Read the model definition and answer for the solid it produces. Units are mm, in the model's axes. A direction names the side the tool comes from. Coordinates: 2 decimals unless noted, no trailing zeros. Loops run counter-clockwise (first coordinate to the right, second up) from the corner with the lowest first, then second, coordinate; pieces in that order, holes last. Notation, with made-up numbers: (46.25, 58.25) -> (50.25, 58.25) arc R19 cw to (50.25, 68.25) -> close; hole circle Ø3 at (-33, 5.5). An arc over 180 degrees is marked (long way). Answer as a JSON object with one key per item and string values. Group by question number.
1) Which of the six approach directions +Z, -Z, +X, -X, +Y, -Y give full straight-line access (tool end or side, diameter ignored) to faces 4 (the face through (12, 11.683, 16)), 5 (the face through (-13, 0, 9)), 6 (the face through (1, -22.892, 10)), 7 (the face through (-4.535, -21, 12))?
2) Section A-A, the plane y = 21 is taken. Give the vertices of the cut face in (x, z).
3) Flat-ended cylindrical pins translate along their axes: P1, Ø4, axis at x = -2.5, y = 0.5, coming from the -Z side; P2, Ø1.5, axis at x = 3, z = 16.5, coming from the +Y side; P3, Ø1.5, axis at x = 8.5, y = 6.5, coming from the +Z side. Find the tip coordinate at first contact, or state that the pin passes through.
4) Determine the mould class of faces 1 (the face through (-14.14, -8.51, 18)), 2 (the face through (0, 29.892, 12)), 3 (the face through (16.253, -28.368, 13.437)) for opening direction Y: released by +Y, released by -Y, zero draft, split by the parting line, or undercut.
5) Section D-D, the plane x = 9 is taken. Give the vertices of the cut face in (y, z) (3 decimals), plus the area to 3 significant figures.
6) Section B-B, the plane x = 16.47 is taken. Give the vertices of the cut face in (y, z).
7) Consider probe 1 along Y at (x, z) = (16.47, 11.8); probe 2 along Y at (x, z) = (5.5, 10.75); probe 3 along Y at (x, z) = (12.5, 9.5) (3 decimals). Determine where each line is inside the solid, lowest interval first. Write a range as [from, to].
8) Section C-C, the plane x = 5 is taken. Give the vertices of the cut face in (y, z), plus the area to 3 significant figures.
from build123d import *

# Parameters (mm, degrees)
SKETCH002_W     = 37.94
SKETCH002_H     = 59.784
SKETCH002_R     = 1
SKETCH002_W_2   = 23.906
SKETCH002_H_2   = 8.634
SKETCH002_W_3   = 11.189
SKETCH002_H_3   = 6.022
SKETCH002_W_4   = 3.58
SKETCH002_H_4   = 8.639
SKETCH002_W_5   = 6.685
SKETCH002_H_5   = 4.785
SKETCH002_W_6   = 7.878
SKETCH002_H_6   = 5.832
PAD_DEPTH       = 9
SKETCH_W        = 27.94
SKETCH_H        = 36.575
SKETCH_H_2      = 12.209
POCKET_DEPTH    = 5
POCKET001_DEPTH = 37.94
SKETCH004_W     = 23.94
SKETCH004_H     = 45.784
POCKET002_DEPTH = 2
SKETCH005_W     = 23.94
SKETCH005_H     = 4
POCKET003_DEPTH = 5
FILLET_R        = 0.75


with BuildPart() as part:
    # Sketch002 → Pad (new body)
    with BuildSketch(Plane.XY.offset(9)):
        Rectangle(SKETCH002_W, SKETCH002_H)
        with Locations((-16.47, 27.392)):
            Circle(SKETCH002_R, mode=Mode.SUBTRACT)
        with Locations((16.47, 27.392)):
            Circle(SKETCH002_R, mode=Mode.SUBTRACT)
        with Locations((-16.47, -27.392)):
            Circle(SKETCH002_R, mode=Mode.SUBTRACT)
        with Locations((16.47, -27.392)):
            Circle(SKETCH002_R, mode=Mode.SUBTRACT)
        with Locations((-0.493, 18.53)):
            Rectangle(SKETCH002_W_2, SKETCH002_H_2, mode=Mode.SUBTRACT)
        with Locations((-2.4905, 7.679)):
            Rectangle(SKETCH002_W_3, SKETCH002_H_3, mode=Mode.SUBTRACT)
        with Locations((7.885, 7.8825)):
            Rectangle(SKETCH002_W_4, SKETCH002_H_4, mode=Mode.SUBTRACT)
        with Locations((9.428, -19.7805)):
            Rectangle(SKETCH002_W_4, SKETCH002_H_4, mode=Mode.SUBTRACT)
        with Locations((9.6625, -9.8675)):
            Rectangle(SKETCH002_W_5, SKETCH002_H_5, mode=Mode.SUBTRACT)
        with Locations((-8.6435, -14.9585)):
            Rectangle(SKETCH002_W_5, SKETCH002_H_5, mode=Mode.SUBTRACT)
        with Locations((-8.121, 1.626)):
            Rectangle(SKETCH002_W_6, SKETCH002_H_6, mode=Mode.SUBTRACT)
        with Locations((-8.474, -20.887)):
            Rectangle(SKETCH002_W_6, SKETCH002_H_6, mode=Mode.SUBTRACT)
    extrude(amount=PAD_DEPTH)

    # Sketch (on Face42 of Pad) → Pocket (cut)
    with BuildSketch(Plane.XY.offset(18)):
        with Locations((0, -6.6045)):
            Rectangle(SKETCH_W, SKETCH_H)
        with Locations((0, 18.7875)):
            Rectangle(SKETCH_W, SKETCH_H_2)
    extrude(amount=-POCKET_DEPTH, mode=Mode.SUBTRACT)

    # Sketch003 → Pocket001 (cut)
    with BuildSketch(Plane(origin=(18.97, 0, 9), x_dir=(0, 1, 0), z_dir=(1, 0, 0))):
        Polygon((12.683, 9), (29.892, 9), (29.892, 5.5), (16.183, 5.5), align=None)
    extrude(amount=-POCKET001_DEPTH, mode=Mode.SUBTRACT)

    # Sketch004 → Pocket002 (cut)
    with BuildSketch(Plane(origin=(0, 0, 9), x_dir=(1, 0, 0), z_dir=(0, 0, -1))):
        Rectangle(SKETCH004_W, SKETCH004_H)
    extrude(amount=-POCKET002_DEPTH, mode=Mode.SUBTRACT)

    # Sketch005 (on Face39 of Pocket002) → Pocket003 (cut)
    with BuildSketch(Plane.XY.offset(18)):
        with Locations((0, -26.892)):
            Rectangle(SKETCH005_W, SKETCH005_H)
    extrude(amount=-POCKET003_DEPTH, mode=Mode.SUBTRACT)

    # Fillet
    fillet_edges = [part.edges().sort_by_distance(p)[0] for p in [
        (-18.97, -29.892, 13.5),
        (18.97, -29.892, 13.5),
        (18.97, 29.892, 11.75),
        (-18.97, 29.892, 11.75),
    ]]
    fillet(fillet_edges, radius=FILLET_R)


solid = part.part
Determined:
{
 "1": {"face 4": "+Z", "face 5": "-Z, +X, -X, +Y, -Y", "face 6": "-Z", "face 7": "+Z, -Z"},
 "2": {"outline": "(-18.97, 9) -> (-12.45, 9) -> (-12.45, 13) -> (-13.97, 13) -> (-13.97, 14.5) -> (-18.97, 14.5) -> close; (11.46, 11) -> (11.97, 11) -> (11.97, 9) -> (18.97, 9) -> (18.97, 14.5) -> (13.97, 14.5) -> (13.97, 13) -> (11.46, 13) -> close"},
 "3": {"P1": "z = 11", "P2": "y = 12.68", "P3": "through"},
 "4": {"face 1": "zero draft", "face 2": "released by +Y", "face 3": "undercut"},
 "5": {"outline": "(-29.892, 9) -> (-24.1, 9) -> (-24.1, 13) -> (-28.892, 13) -> (-28.892, 18) -> (-29.892, 18) -> close; (-15.461, 11) -> (-12.26, 11) -> (-12.26, 13) -> (-15.461, 13) -> close; (-7.475, 11) -> (3.563, 11) -> (3.563, 13) -> (-7.475, 13) -> close; (12.202, 11) -> (14.213, 11) -> (14.213, 13) -> (12.683, 13) -> (12.683, 18) -> (12.202, 18) -> close; (22.847, 11) -> (22.892, 11) -> (22.892, 9) -> (29.892, 9) -> (29.892, 14.5) -> (24.892, 14.5) -> (24.892, 13) -> (22.847, 13) -> close", "area": "98.7 mm²"},
 "6": {"outline": "(-29.89, 9) -> (-28.39, 9) -> (-28.39, 18) -> (-29.89, 18) -> close; (-26.39, 9) -> (26.39, 9) -> (26.39, 14.5) -> (16.18, 14.5) -> (12.68, 18) -> (-26.39, 18) -> close; (28.39, 9) -> (29.89, 9) -> (29.89, 14.5) -> (28.39, 14.5) -> close"},
 "7": {"probe 1": "[-29.89, -28.39], [-26.39, 26.39], [28.39, 29.89]", "probe 2": "[-29.89, -22.89], [22.89, 29.89]", "probe 3": "[-29.892, -12.26], [-7.475, 29.892]"},
 "8": {"outline": "(-29.89, 9) -> (-22.89, 9) -> (-22.89, 11) -> (14.21, 11) -> (14.21, 13) -> (12.68, 13) -> (12.68, 18) -> (11.68, 18) -> (11.68, 13) -> (-28.89, 13) -> (-28.89, 18) -> (-29.89, 18) -> close; (22.85, 11) -> (22.89, 11) -> (22.89, 9) -> (29.89, 9) -> (29.89, 14.5) -> (24.89, 14.5) -> (24.89, 13) -> (22.85, 13) -> close", "area": "148 mm²"}
}
